Verification items for the finished model (mm, model axes). Round coordinates to 2 decimals unless told otherwise and drop trailing zeros. Write each loop counter-clockwise with the first axis right and the second up, starting at its lowest first coordinate (ties: lowest second). Pieces come first, ordered by that corner, then holes. Notation, with made-up numbers: (71, 76) - (118, 76) arc R15 ccw to (118, 91) - close; hole circle Ø1 at (74.5, -26). An arc over 180 degrees is marked (long way). Answer as a JSON object with one key per item and string values. Group by question number.
1) Section check D-D (z = 0). Enter the section's corners in (x, y), then the cut area to 3 significant figures.
2) Section check A-A (z = 30). Enter the section's corners in (x, y).
3) Mould release check, pull along X, two halves, no side actions. Record for faces 1 (the flat face through (25, 10, 13)), 2 (the cylindrical face through (-6, 10, 0)), 3 (the flat face through (-25, 10, 13)): +X half, -X half, draft (parallel to the pull), parting line (faces both ways), or undercut.
4) Section check C-C (y = 13). Enter the section's corners in (x, z), then the cut area to 3 significant figures.
5) Section check B-B (x = 0). Enter the section's corners in (y, z).
6) Thickness scan on line 1 (Z direction, x = 0, y = 11.25); line 2 (X direction, y = 5, z = 30); line 3 (X direction, y = 12.75, z = 5.5). Record the ranges inside material, lowest first.
7) Go/stop test with a flat-tipped pin: pin 1 Ø8 at (x, z) = (-1, 27) entering from +Y. Record where the tip stops, or that it passes through.
```python
from build123d import *

# Parameters (mm, degrees)
SKETCH1_W           = 50
SKETCH1_H           = 75
SKETCH1_R           = 6
SKETCH1_R_2         = 8
BOSS_EXTRUDE1_DEPTH = 20


with BuildPart() as part:
    # Sketch1 → Boss-Extrude1 (new body)
    with BuildSketch(Plane(origin=(0, 0, 0), x_dir=(1, 0, 0), z_dir=(0, 1, 0))):
        with Locations((0, -12.5)):
            Rectangle(SKETCH1_W, SKETCH1_H)
        Circle(SKETCH1_R, mode=Mode.SUBTRACT)
        with Locations((0, -30)):
            Circle(SKETCH1_R_2, mode=Mode.SUBTRACT)
    extrude(amount=BOSS_EXTRUDE1_DEPTH)


solid = part.part
```
Returned:
{
 "1": {"outline": "(-25, 0) - (-6, 0) - (-6, 20) - (-25, 20) - close; (6, 0) - (25, 0) - (25, 20) - (6, 20) - close", "area": "760 mm2"},
 "2": {"outline": "(-25, 0) - (-8, 0) - (-8, 20) - (-25, 20) - close; (8, 0) - (25, 0) - (25, 20) - (8, 20) - close"},
 "3": {"face 1": "+X half", "face 2": "undercut", "face 3": "-X half"},
 "4": {"outline": "(-25, -25) - (25, -25) - (25, 50) - (-25, 50) - close; hole circle Ø16 at (0, 30); hole circle Ø12 at (0, 0)", "area": "3,440 mm2"},
 "5": {"outline": "(0, -25) - (20, -25) - (20, -6) - (0, -6) - close; (0, 6) - (20, 6) - (20, 22) - (0, 22) - close; (0, 38) - (20, 38) - (20, 50) - (0, 50) - close"},
 "6": {"line 1": "-25 to -6, 6 to 22, 38 to 50", "line 2": "-25 to -8, 8 to 25", "line 3": "-25 to -2.4, 2.4 to 25"},
 "7": {"pin 1": "through"}
}
